Source: CAD feature listing. Evaluate the final solid. Frame: model axes, mm. A direction names the side the tool comes from. Coordinates: 2 decimals unless noted, no trailing zeros. Write each loop counter-clockwise with the first axis right and the second up, starting at its lowest first coordinate (ties: lowest second). Pieces come first, ordered by that corner, then holes. Notation, with made-up numbers: M 67,-30 L 106,-30 A18 cw 106,-11 Z; hole C 0.25,83 d2. An arc over 180 degrees is marked long. Answer as CSV lines item,"result". Start each with the question number.
1. Contact query for flat-ended pins moving along their axis: pin 1 Ø4 at (y, z) = (-2, 6.5) entering from -X; pin 2 Ø3 at (x, z) = (24, 4.5) entering from +Y; pin 3 Ø2.5 at (x, z) = (23.5, 4.5) entering from -Y; pin 4 Ø4 at (x, y) = (9, 16.5) entering from +Z. Output: stop coordinate, or through.
2. Section D-D on z = 12.5. Return the cut outline in (x, y).
3. Section A-A on z = 2. Return the cut outline in (x, y) (3 decimals), plus the area to 3 significant figures.
4. Line query: probe 1 along Y at (x, z) = (22, 8.75); probe 2 along Z at (x, y) = (57.5, -26.25) (3 decimals); probe 3 along Y at (x, z) = (-2, 8.25). Output: solid intervals per line, ascending. Write a range as [from, to].
5. Section B-B on x = 59.5. Return the cut outline in (y, z) (3 decimals).
6. Reachability of faces 4 (the face through (24, 3.084, 5)), 5 (the face through (61.963, -23, 7)), 6 (the face through (-9.75, 0, 7)) from +Z, -Z, +X, -X, +Y, -Y: full face, straight path, thin tool, end or side. Return the list, or none.
7. Section C-C on y = -15. Return the cut outline in (x, z), plus the area to 3 significant figures.
8. Mould query, pull axis X, two halves, no side actions, for faces 1 (the face through (61.963, 24, 8.4)), 2 (the face through (-17.65, 0.75, 4.44)), 3 (the face through (15, 0, 9)). Classes: pulls with the +X half, pulls with the -X half, needs draft (parallel to the pull), parting line crosses it, or undercut.
```python
from build123d import *

# Parameters (mm, degrees)
F0_R           = 7.875
F1_DEPTH       = 9
F2_R           = 7.875
F3_DEPTH       = 4.8
F4_DEPTH       = 15
F5_R           = 5
F8_D           = 4.5
F8_DEPTH       = 25
F8_CBORE_D     = 8.25
F8_CBORE_DEPTH = 17
F8_TIP         = 1.3519363928
F11_DEPTH      = 25


# Not quite as in the source:
# - two fillets or chamfers of one size are made in one step


with BuildPart() as f1:
    # F0 (on Top) → F1 (new body)
    with BuildSketch(Plane.XY):
        with BuildLine():
            ThreePointArc((13.8549873727, 10.4671236312), (-17.6653132634, 0.1978340536), (13.609496128, -10.7964352789))
            Line((13.609496128, -10.7964352789), (41.3727938251, -10.7964352789))
            ThreePointArc((41.3727938251, -10.7964352789), (39.3632549532, -0.1760847087), (41.2479854227, 10.4671236312))
            Line((41.2479854227, 10.4671236312), (13.8549873727, 10.4671236312))
        make_face()
        Circle(F0_R, mode=Mode.SUBTRACT)
        with BuildLine():
            ThreePointArc((41.2479854227, 10.4671236312), (39.3632549532, -0.1760847087), (41.3727938251, -10.7964352789))
            ThreePointArc((41.3727938251, -10.7964352789), (52.3906001106, -24.7375530153), (69.362738185, -30))
            Line((69.362738185, -30), (69.362738185, -22.5))
            ThreePointArc((69.362738185, -22.5), (46.862738185, 0), (69.362738185, 22.5))
            Line((69.362738185, 22.5), (69.362738185, 30))
            ThreePointArc((69.362738185, 30), (52.2456956387, 24.6375090963), (41.2479854227, 10.4671236312))
        make_face()
    extrude(amount=F1_DEPTH)

    # F2 (on face) → F3 (cut)
    with BuildSketch(Plane.XY.offset(9)):
        Polygon((9.75, -5.6291651246), (9.75, 5.6291651246), (0, 11.2583302492), (-9.75, 5.6291651246), (-9.75, -5.6291651246), (0, -11.2583302492), align=None)
        Circle(F2_R, mode=Mode.SUBTRACT)
    extrude(amount=-F3_DEPTH, mode=Mode.SUBTRACT)

    # F0 (on Top) → F4 (join)
    with BuildSketch(Plane.XY):
        with BuildLine():
            ThreePointArc((41.2479854227, 10.4671236312), (39.3632549532, -0.1760847087), (41.3727938251, -10.7964352789))
            ThreePointArc((41.3727938251, -10.7964352789), (52.3906001106, -24.7375530153), (69.362738185, -30))
            Line((69.362738185, -30), (69.362738185, -22.5))
            ThreePointArc((69.362738185, -22.5), (46.862738185, 0), (69.362738185, 22.5))
            Line((69.362738185, 22.5), (69.362738185, 30))
            ThreePointArc((69.362738185, 30), (52.2456956387, 24.6375090963), (41.2479854227, 10.4671236312))
        make_face()
    extrude(amount=F4_DEPTH)

    # F5
    f5_edges = [f1.edges().sort_by_distance(p)[0] for p in [
        (13.609496, -10.796435, 4.5),
        (41.247985, 10.467124, 4.5),
        (41.372794, -10.796435, 4.5),
        (39.363255, -0.176085, 9),
        (13.854987, 10.467124, 4.5),
        (69.362738, -22.5, 7.5),
        (69.362738, 22.5, 7.5),
    ]]
    fillet(f5_edges, radius=F5_R)

    # F8
    with Locations(Plane(origin=(44.962738185, 0, 0), x_dir=(0, 1, 0), z_dir=(-1, 0, 0))):
        with Locations((26.25, -7.5), (-26.25, -7.5)):
            CounterBoreHole(F8_D / 2, F8_CBORE_D / 2, F8_CBORE_DEPTH, depth=F8_DEPTH)
            with Locations((0, 0, -(F8_DEPTH + F8_TIP / 2))):  # 118° drill point
                Cone(0, F8_D / 2, F8_TIP, mode=Mode.SUBTRACT)

    # F10 (on face) → F11 (cut)
    with BuildSketch(Plane.XY.offset(9)):
        with BuildLine():
            ThreePointArc((19.4264538586, 5.0838164277), (18.4264538586, 4.0838164277), (19.4264538586, 3.0838164277))
            Line((19.4264538586, 3.0838164277), (28.1441677362, 3.0838164277))
            ThreePointArc((28.1441677362, 3.0838164277), (29.1441677362, 4.0838164277), (28.1441677362, 5.0838164277))
            Line((28.1441677362, 5.0838164277), (19.4264538586, 5.0838164277))
        make_face()
        with BuildLine():
            Line((28.1441677362, -3.0838164277), (19.4264538586, -3.0838164277))
            ThreePointArc((19.4264538586, -3.0838164277), (18.4264538586, -4.0838164277), (19.4264538586, -5.0838164277))
            Line((19.4264538586, -5.0838164277), (28.1441677362, -5.0838164277))
            ThreePointArc((28.1441677362, -5.0838164277), (29.1441677362, -4.0838164277), (28.1441677362, -3.0838164277))
        make_face()
    extrude(amount=-F11_DEPTH, mode=Mode.SUBTRACT)


solid = f1.part
```
Values:
1,pin 1,"x = -17.67"
1,pin 2,"y = 10.47"
1,pin 3,"y = -10.8"
1,pin 4,"z = 9"
2,outline,"M 41.66,12.09 A30.23 ccw 41.79,-12.39 A5 cw 42.59,-13.54 A30 ccw 69.36,-30 L 69.36,-27.04 A5 ccw 65.27,-22.12 A22.5 cw 65.27,22.12 A5 ccw 69.36,27.04 L 69.36,30 A30 ccw 42.45,13.26 A5 cw Z"
3,outline,"M 12.299,-12.287 A5 cw 15.86,-10.796 L 38.13,-10.796 A5 cw 42.592,-13.54 A30 ccw 69.363,-30 L 69.363,-27.042 A5 ccw 65.272,-22.125 A22.5 cw 65.272,22.125 A5 ccw 69.363,27.042 L 69.363,30 A30 ccw 42.451,13.258 A5 cw 37.966,10.467 L 16.17,10.467 A5 cw 12.54,12.029 A17.5 ccw long Z; hole C 0,0 d15.75; hole M 19.426,-5.084 L 28.144,-5.084 A1 ccw 28.144,-3.084 L 19.426,-3.084 A1 ccw Z; hole M 19.426,3.084 L 28.144,3.084 A1 ccw 28.144,5.084 L 19.426,5.084 A1 ccw Z"
3,area,"1,850 mm²"
4,probe 1,"[-10.8, -5.08], [-3.08, 3.08], [5.08, 10.47]"
4,probe 2,"[0, 3.375], [11.625, 15]"
4,probe 3,"[-17.41, -10.1], [10.1, 17.4]"
5,outline,"M -28.332,0 L -20.223,0 L -20.223,15 L -28.332,15 L -28.332,11.061 A4.125 cw long -28.332,3.939 Z; M 20.223,0 L 28.332,0 L 28.332,3.939 A4.125 cw long 28.332,11.061 L 28.332,15 L 20.223,15 Z"
6,face 4,"+Z, -Z"
6,face 5,"-X"
6,face 6,"+Z"
7,outline,"M -9.19,0 L 8.85,0 L 8.85,9 L -9.19,9 Z; M 43.38,0 L 52.59,0 L 52.59,15 L 43.38,15 Z"
7,area,"301 mm²"
8,face 1,"pulls with the -X half"
8,face 2,"undercut"
8,face 3,"needs draft"
